```python
from build123d import *

# Parameters (mm, degrees)
ESQUISSE2_W                  = 261.4
ESQUISSE2_H                  = 50
BOSS_EXTRU_1_DEPTH           = 42
ENL_V_MAT_EXTRU_1_DEPTH      = 270.432663202
ENL_V_MAT_EXTRU_1_DEPTH_BACK = 20


with BuildPart() as part:
    # Esquisse2 → Boss.-Extru.1 (new body)
    with BuildSketch(Plane.XY):
        with Locations((130.7, 25)):
            Rectangle(ESQUISSE2_W, ESQUISSE2_H)
    extrude(amount=BOSS_EXTRU_1_DEPTH)

    # Esquisse3 → Enlèv. mat.-Extru.1 (cut, two sides: drawn at the far end of the back side and taken through both)
    with BuildSketch(Plane.XY.offset(42).offset(-ENL_V_MAT_EXTRU_1_DEPTH_BACK)):
        Polygon((-536.231736025, 20), (0, 20), (261.4, 20), (797.631736025, 20), (797.631736025, 1092.46347205), (-536.231736025, 1092.46347205), align=None)
    extrude(amount=ENL_V_MAT_EXTRU_1_DEPTH + ENL_V_MAT_EXTRU_1_DEPTH_BACK, mode=Mode.SUBTRACT)


solid = part.part
```
Model file for the job. Use its own axes, mm. A direction names the side the tool comes from. Coordinates: 2 decimals unless noted, no trailing zeros. Write each loop counter-clockwise with the first axis right and the second up, starting at its lowest first coordinate (ties: lowest second). Pieces come first, ordered by that corner, then holes. Notation, with made-up numbers: (5.25, 38) - (27.25, 38) arc R27 cw to (27.25, 64) - close; hole circle Ø6 at (75.5, -11.75). An arc over 180 degrees is marked (long way). One line per item, written item: value. Start each with the question number.
1. Slice it at B-B (y = 25). Write the cut outline in (x, z).
2. Probe line 1 (Y direction, x = 139.5, z = 37); line 2 (Z direction, x = 33.5, y = 21). List the from-to ranges inside material, lowest first. Write a range as from..to.
3. Slice it at C-C (z = 34). Write the cut outline in (x, y).
4. Flat gauge pins, fed straight in: pin 1 (9 mm diameter, centred on x = 166, y = 41, fed in from +Z); pin 2 (10 mm diameter, centred on x = 169, z = 27.5, fed in from +Y); pin 3 (2 mm diameter, centred on x = 215, z = 33, fed in from -Y). Where does each tip first touch, or does it go through?
5. Tool access for faces 1 (the flat face through (129, 0, 21)), 2 (the flat face through (129, 35, 22)): list every direction of +Z, -Z, +X, -X, +Y, -Y with a clear straight run to the whole face (end or side of a thin tool).
6. Slice it at A-A (x = 158). Write the cut outline in (y, z).
Answers below:
1. outline: (0, 0) - (261.4, 0) - (261.4, 22) - (0, 22) - close
2. line 1: y = 0..20
2. line 2: z = 0..22
3. outline: (0, 0) - (261.4, 0) - (261.4, 20) - (0, 20) - close
4. pin 1: stops at z = 22
4. pin 2: stops at y = 20
4. pin 3: stops at y = 0
5. face 1: +Z, -Z, +X, -X, -Y
5. face 2: +Z, +X, -X, +Y
6. outline: (0, 0) - (50, 0) - (50, 22) - (20, 22) - (20, 42) - (0, 42) - close
